Here's how the part is built. I have some questions about the finished solid (model axes, mm). Face numbers are marked on the shaded views. Round coordinates to 2 decimals unless told otherwise and drop trailing zeros. Loops run counter-clockwise (first coordinate to the right, second up) from the corner with the lowest first, then second, coordinate; pieces in that order, holes last. Notation, with made-up numbers: M -39.75,88.5 L -24.75,88.5 A16 ccw -24.75,112.5 Z; hole C 53,14 d2. An arc over 180 degrees is marked long. Use a Markdown table: item, result.
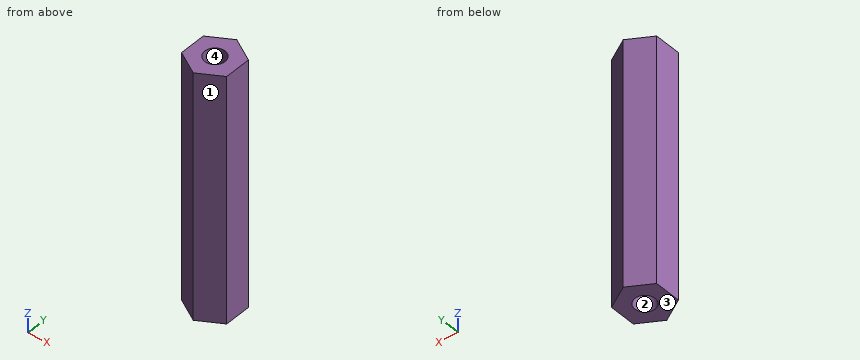
Autodesk Inventor part; units mm, degrees
ref_plane "YZ Plane" through (0, 0, 0) normal (1, 0, 0) x (0, 1, 0)
ref_plane "XZ Plane" through (0, 0, 0) normal (0, 1, 0) x (-1, 0, 0)
ref_plane "XY Plane" through (0, 0, 0) normal (0, 0, 1) x (1, 0, 0)
sketch "スケッチ1" plane through (0, 0, 0) normal (0, 0, 1) x (1, 0, 0)
  line L0 (0, 3.1754) -> (2.75, 1.5877)
  line L1 (2.75, 1.5877) -> (2.75, -1.5877)
  line L2 (2.75, -1.5877) -> (0, -3.1754)
  line L3 (0, -3.1754) -> (-2.75, -1.5877)
  line L4 (-2.75, -1.5877) -> (-2.75, 1.5877)
  line L5 (-2.75, 1.5877) -> (0, 3.1754)
  point P0 (0, 0)
  point P1 (0, 0)
  dimension "d0" = 5.5
extrude "押し出し1" add sketch "スケッチ1" along normal blind 30
sketch "スケッチ2" plane through (0, 0, 30) normal (0, 0, 1) x (1, 0, 0)
  line L0 (2.75, 1.5877) -> (0, 3.1754)
  line L1 (0, 3.1754) -> (-2.75, 1.5877)
  line L2 (-2.75, 1.5877) -> (-2.75, -1.5877)
  line L3 (-2.75, -1.5877) -> (0, -3.1754)
  line L4 (0, -3.1754) -> (2.75, -1.5877)
  line L5 (2.75, -1.5877) -> (2.75, 1.5877)
  point P0 (0, 0)
hole "穴1" at (0, 0, 30) direction (0, 0, -1) diameter 2.459 depth 8.8 tip angle 118
sketch "スケッチ3" plane through (0, 0, 0) normal (0, 0, -1) x (-1, 0, 0)
  line L0 (0, 3.1754) -> (-2.75, 1.5877)
  line L1 (-2.75, 1.5877) -> (-2.75, -1.5877)
  line L2 (-2.75, -1.5877) -> (0, -3.1754)
  line L3 (0, -3.1754) -> (2.75, -1.5877)
  line L4 (2.75, -1.5877) -> (2.75, 1.5877)
  line L5 (2.75, 1.5877) -> (0, 3.1754)
  point P0 (0, 0)
hole "穴2" at (0, 0, 0) direction (0, 0, 1) diameter 2.459 depth 8.8 tip angle 118
properties part number "黄銅スペーサー（六角）_ASB-330E" material "真鍮、ソフト イエロー"
1. Imagine slicing it at B-B, the plane x = -1.8. Write out the boundary of the cut face in (y, z).
Answer sheet:
| item | result |
|---|---|
| outline | M -2.14,0 L 2.14,0 L 2.14,30 L -2.14,30 Z |
2. We'd pull the mould along X, two halves only. Please class the marked faces 1, 2, 3 and 4: +X half, -X half, draft (parallel to the pull), parting line (faces both ways), or undercut.
Answer sheet:
| item | result |
|---|---|
| face 1 | +X half |
| face 2 | undercut |
| face 3 | draft |
| face 4 | undercut |
3. For pin 1 Ø1.5 at (x, y) = (0, 0) entering from -Z; pin 2 Ø2 at (x, y) = (0, 0) entering from +Z; pin 3 Ø1.5 at (x, z) = (1.5, 23.5) entering from -Y, each with a flat end and sliding along its axis, tell me the tip position at first contact or that it passes through.
Answer sheet:
| item | result |
|---|---|
| pin 1 | z = 9.09 |
| pin 2 | z = 21.06 |
| pin 3 | y = -2.74 |
4. Imagine slicing it at C-C, the plane x = 2.05. Write out the boundary of the cut face in (y, z), then the cut area to 3 significant figures.
Answer sheet:
| item | result |
|---|---|
| outline | M -1.99,0 L 1.99,0 L 1.99,30 L -1.99,30 Z |
| area | 120 mm2 |
5. Imagine slicing it at A-A, the plane z = 3.5. Write out the boundary of the cut face in (x, y), then the cut area to 3 significant figures.
Answer sheet:
| item | result |
|---|---|
| outline | M -2.75,-1.59 L 0,-3.18 L 2.75,-1.59 L 2.75,1.59 L 0,3.18 L -2.75,1.59 Z; hole C 0,0 d2.46 |
| area | 21.4 mm2 |
6. I need wall thicknesses on probe 1 along X at (y, z) = (0, 28.25); probe 2 along Y at (x, z) = (-0.45, 25.5); probe 3 along X at (y, z) = (-2.75, 24.25). Which ranges of each line are inside material? Lowest first, please. Write a range as from..to.
Answer sheet:
| item | result |
|---|---|
| probe 1 | -2.75..-1.23, 1.23..2.75 |
| probe 2 | -2.92..-1.14, 1.14..2.92 |
| probe 3 | -0.74..0.74 |
